Check sheet for the modelled part. Datum: model origin and axes. Units: mm. Face numbers are marked on the shaded views. Give positions to 0.01 mm unless a question says otherwise; leave off trailing zeros.
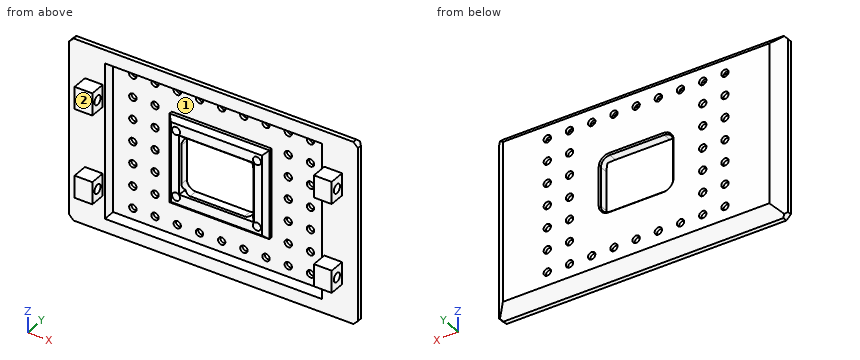
```python
from build123d import *

# Parameters (mm, degrees)
SKETCH1_W           = 130
SKETCH1_H           = 82
BOSS_EXTRUDE1_DEPTH = 2
CHAMFER2_SIZE       = 2
SKETCH4_W           = 8
SKETCH4_H           = 10
BOSS_EXTRUDE2_DEPTH = 7
SKETCH5_R           = 2.05
CUT_EXTRUDE1_DEPTH  = 130.747485656
SKETCH6_W           = 97.8
SKETCH6_H           = 70
CUT_EXTRUDE2_DEPTH  = 5.5
SKETCH7_R           = 1.65
CUT_EXTRUDE3_DEPTH  = 78.860452228
SKETCH10_W          = 50
SKETCH10_H          = 50
BOSS_EXTRUDE3_DEPTH = 1.5
SKETCH11_W          = 45
SKETCH11_H          = 40
BOSS_EXTRUDE4_DEPTH = 3.5
SKETCH12_R          = 1.35
SKETCH12_W          = 32.5
SKETCH12_H          = 25.5
CUT_EXTRUDE4_DEPTH  = 79.115299533
CHAMFER3_SIZE       = 0.6
FILLET1_R           = 4
CHAMFER4_SIZE       = 0.6
SKETCH13_R          = 1.35
BOSS_EXTRUDE5_DEPTH = 1
SKETCH14_R          = 1.8
CUT_EXTRUDE5_DEPTH  = 4
CHAMFER5_SIZE       = 2


with BuildPart() as part:
    # Sketch1 → Boss-Extrude1 (new body)
    with BuildSketch(Plane(origin=(0, 0, 0), x_dir=(1, 0, 0), z_dir=(0, 1, 0))):
        Rectangle(SKETCH1_W, SKETCH1_H)
    extrude(amount=BOSS_EXTRUDE1_DEPTH)

    # Sketch3 → Loft1 section 0
    with BuildSketch(Plane(origin=(0, 7, 0), x_dir=(1, 0, 0), z_dir=(0, 1, 0))):
        with BuildLine():
            Line((-60, -36), (60, -36))
            Line((60, -36), (60, 36))
            Line((60, 36), (-60, 36))
            Line((-60, 36), (-60, -36))
        make_face()
    # Sketch2 → Loft1 section 1
    with BuildSketch(Plane(origin=(0, 2, 0), x_dir=(1, 0, 0), z_dir=(0, 1, 0))):
        with BuildLine():
            Line((65, -41), (65, 41))
            Line((65, 41), (-65, 41))
            Line((-65, 41), (-65, -41))
            Line((-65, -41), (65, -41))
        make_face()
    loft()

    # Chamfer2
    chamfer2_edges = [part.edges().sort_by_distance(p)[0] for p in [
        (65, 1, 41),
        (-65, 1, 41),
        (-65, 1, -41),
        (65, 1, -41),
    ]]
    chamfer(chamfer2_edges, length=CHAMFER2_SIZE)

    # Sketch4 → Boss-Extrude2 (add)
    with BuildSketch(Plane.XZ):
        with Locations((-53.9, 20)):
            Rectangle(SKETCH4_W, SKETCH4_H)
        with Locations((-53.9, -20)):
            Rectangle(SKETCH4_W, SKETCH4_H)
        with Locations((53.9, -20)):
            Rectangle(SKETCH4_W, SKETCH4_H)
        with Locations((53.9, 20)):
            Rectangle(SKETCH4_W, SKETCH4_H)
    extrude(amount=BOSS_EXTRUDE2_DEPTH)

    # Sketch5 → Cut-Extrude1 (cut, through all)
    with BuildSketch(Plane.ZY.offset(57.9)):
        with Locations((-20, -3.5)):
            Circle(SKETCH5_R)
        with Locations((20, -3.5)):
            Circle(SKETCH5_R)
    extrude(amount=-CUT_EXTRUDE1_DEPTH, mode=Mode.SUBTRACT)

    # Sketch6 → Cut-Extrude2 (cut)
    with BuildSketch(Plane.XZ):
        Rectangle(SKETCH6_W, SKETCH6_H)
    extrude(amount=-CUT_EXTRUDE2_DEPTH, mode=Mode.SUBTRACT)

    # Sketch7 → Cut-Extrude3 (cut, through all)
    with BuildSketch(Plane.XZ.offset(-5.5)):
        with Locations(Location((0, 0, 0), (0, 0, 270))):
            Circle(SKETCH7_R)
        with Locations(Location((10, 0, 0), (0, 0, 270))):
            Circle(SKETCH7_R)
        with Locations(Location((20, 0, 0), (0, 0, 270))):
            Circle(SKETCH7_R)
        with Locations(Location((30, 0, 0), (0, 0, 270))):
            Circle(SKETCH7_R)
        with Locations(Location((40, 0, 0), (0, 0, 270))):
            Circle(SKETCH7_R)
        with Locations(Location((10, 10, 0), (0, 0, 270))):
            Circle(SKETCH7_R)
        with Locations(Location((20, 10, 0), (0, 0, 270))):
            Circle(SKETCH7_R)
        with Locations(Location((30, 10, 0), (0, 0, 270))):
            Circle(SKETCH7_R)
        with Locations(Location((40, 10, 0), (0, 0, 270))):
            Circle(SKETCH7_R)
        with Locations(Location((10, 20, 0), (0, 0, 270))):
            Circle(SKETCH7_R)
        with Locations(Location((20, 20, 0), (0, 0, 270))):
            Circle(SKETCH7_R)
        with Locations(Location((30, 20, 0), (0, 0, 270))):
            Circle(SKETCH7_R)
        with Locations(Location((40, 20, 0), (0, 0, 270))):
            Circle(SKETCH7_R)
        with Locations(Location((10, 30, 0), (0, 0, 270))):
            Circle(SKETCH7_R)
        with Locations(Location((20, 30, 0), (0, 0, 270))):
            Circle(SKETCH7_R)
        with Locations(Location((30, 30, 0), (0, 0, 270))):
            Circle(SKETCH7_R)
        with Locations(Location((40, 30, 0), (0, 0, 270))):
            Circle(SKETCH7_R)
        with Locations(Location((0, 10, 0), (0, 0, 270))):
            Circle(SKETCH7_R)
        with Locations(Location((0, 20, 0), (0, 0, 270))):
            Circle(SKETCH7_R)
        with Locations(Location((0, 30, 0), (0, 0, 270))):
            Circle(SKETCH7_R)
        with Locations(Location((-40, 30, 0), (0, 0, 270))):
            Circle(SKETCH7_R)
        with Locations(Location((-30, 30, 0), (0, 0, 270))):
            Circle(SKETCH7_R)
        with Locations(Location((-20, 30, 0), (0, 0, 270))):
            Circle(SKETCH7_R)
        with Locations(Location((-10, 30, 0), (0, 0, 270))):
            Circle(SKETCH7_R)
        with Locations(Location((-40, 20, 0), (0, 0, 270))):
            Circle(SKETCH7_R)
        with Locations(Location((-30, 20, 0), (0, 0, 270))):
            Circle(SKETCH7_R)
        with Locations(Location((-20, 20, 0), (0, 0, 270))):
            Circle(SKETCH7_R)
        with Locations(Location((-10, 20, 0), (0, 0, 270))):
            Circle(SKETCH7_R)
        with Locations(Location((-40, 10, 0), (0, 0, 270))):
            Circle(SKETCH7_R)
        with Locations(Location((-30, 10, 0), (0, 0, 270))):
            Circle(SKETCH7_R)
        with Locations(Location((-20, 10, 0), (0, 0, 270))):
            Circle(SKETCH7_R)
        with Locations(Location((-10, 10, 0), (0, 0, 270))):
            Circle(SKETCH7_R)
        with Locations(Location((-40, 0, 0), (0, 0, 270))):
            Circle(SKETCH7_R)
        with Locations(Location((-30, 0, 0), (0, 0, 270))):
            Circle(SKETCH7_R)
        with Locations(Location((-20, 0, 0), (0, 0, 270))):
            Circle(SKETCH7_R)
        with Locations(Location((-10, 0, 0), (0, 0, 270))):
            Circle(SKETCH7_R)
        with Locations(Location((-10, -10, 0), (0, 0, 270))):
            Circle(SKETCH7_R)
        with Locations(Location((-20, -10, 0), (0, 0, 270))):
            Circle(SKETCH7_R)
        with Locations(Location((-30, -10, 0), (0, 0, 270))):
            Circle(SKETCH7_R)
        with Locations(Location((-40, -10, 0), (0, 0, 270))):
            Circle(SKETCH7_R)
        with Locations(Location((-10, -20, 0), (0, 0, 270))):
            Circle(SKETCH7_R)
        with Locations(Location((-20, -20, 0), (0, 0, 270))):
            Circle(SKETCH7_R)
        with Locations(Location((-30, -20, 0), (0, 0, 270))):
            Circle(SKETCH7_R)
        with Locations(Location((-40, -20, 0), (0, 0, 270))):
            Circle(SKETCH7_R)
        with Locations(Location((-10, -30, 0), (0, 0, 270))):
            Circle(SKETCH7_R)
        with Locations(Location((-20, -30, 0), (0, 0, 270))):
            Circle(SKETCH7_R)
        with Locations(Location((-30, -30, 0), (0, 0, 270))):
            Circle(SKETCH7_R)
        with Locations(Location((-40, -30, 0), (0, 0, 270))):
            Circle(SKETCH7_R)
        with Locations(Location((0, -30, 0), (0, 0, 270))):
            Circle(SKETCH7_R)
        with Locations(Location((0, -20, 0), (0, 0, 270))):
            Circle(SKETCH7_R)
        with Locations(Location((0, -10, 0), (0, 0, 270))):
            Circle(SKETCH7_R)
        with Locations(Location((40, -30, 0), (0, 0, 270))):
            Circle(SKETCH7_R)
        with Locations(Location((30, -30, 0), (0, 0, 270))):
            Circle(SKETCH7_R)
        with Locations(Location((20, -30, 0), (0, 0, 270))):
            Circle(SKETCH7_R)
        with Locations(Location((10, -30, 0), (0, 0, 270))):
            Circle(SKETCH7_R)
        with Locations(Location((40, -20, 0), (0, 0, 270))):
            Circle(SKETCH7_R)
        with Locations(Location((30, -20, 0), (0, 0, 270))):
            Circle(SKETCH7_R)
        with Locations(Location((20, -20, 0), (0, 0, 270))):
            Circle(SKETCH7_R)
        with Locations(Location((10, -20, 0), (0, 0, 270))):
            Circle(SKETCH7_R)
        with Locations(Location((40, -10, 0), (0, 0, 270))):
            Circle(SKETCH7_R)
        with Locations(Location((30, -10, 0), (0, 0, 270))):
            Circle(SKETCH7_R)
        with Locations(Location((20, -10, 0), (0, 0, 270))):
            Circle(SKETCH7_R)
        with Locations(Location((10, -10, 0), (0, 0, 270))):
            Circle(SKETCH7_R)
    extrude(amount=-CUT_EXTRUDE3_DEPTH, mode=Mode.SUBTRACT)

    # Sketch10 → Boss-Extrude3 (add)
    with BuildSketch(Plane(origin=(0, 7, 0), x_dir=(1, 0, 0), z_dir=(0, 1, 0))):
        Rectangle(SKETCH10_W, SKETCH10_H)
    extrude(amount=-BOSS_EXTRUDE3_DEPTH)

    # Sketch11 → Boss-Extrude4 (add)
    with BuildSketch(Plane.XZ.offset(-5.5)):
        Rectangle(SKETCH11_W, SKETCH11_H)
    extrude(amount=BOSS_EXTRUDE4_DEPTH)

    # Sketch12 → Cut-Extrude4 (cut, through all)
    with BuildSketch(Plane(origin=(0, 7, 0), x_dir=(1, 0, 0), z_dir=(0, 1, 0))):
        with Locations(Location((-18.21, 14.785, 0), (0, 0, 270))):
            Circle(SKETCH12_R)
        with Locations(Location((18.21, 14.785, 0), (0, 0, 270))):
            Circle(SKETCH12_R)
        with Locations(Location((18.21, -14.785, 0), (0, 0, 270))):
            Circle(SKETCH12_R)
        with Locations(Location((-18.21, -14.785, 0), (0, 0, 270))):
            Circle(SKETCH12_R)
        Rectangle(SKETCH12_W, SKETCH12_H)
    extrude(amount=-CUT_EXTRUDE4_DEPTH, mode=Mode.SUBTRACT)

    # Chamfer3
    chamfer3_edges = [part.edges().sort_by_distance(p)[0] for p in [
        (0, 2, -12.75),
        (-16.25, 2, 0),
        (0, 2, 12.75),
        (16.25, 2, 0),
    ]]
    chamfer(chamfer3_edges, length=CHAMFER3_SIZE)

    # Fillet1
    fillet1_edges = [part.edges().sort_by_distance(p)[0] for p in [
        (-16.25, 4.8, 12.75),
        (16.25, 4.8, 12.75),
        (16.25, 4.8, -12.75),
        (-16.25, 4.8, -12.75),
    ]]
    fillet(fillet1_edges, radius=FILLET1_R)

    # Chamfer4
    chamfer4_edges = [part.edges().sort_by_distance(p)[0] for p in [
        (16.25, 7, 0),
        (0, 7, 12.75),
        (-16.25, 7, 0),
        (0, 7, -12.75),
        (15.078427125, 7, 11.578427125),
        (-15.078427125, 7, 11.578427125),
        (15.078427125, 7, -11.578427125),
        (-15.078427125, 7, -11.578427125),
    ]]
    chamfer(chamfer4_edges, length=CHAMFER4_SIZE)

    # Sketch13 → Boss-Extrude5 (add)
    with BuildSketch(Plane(origin=(0, 7, 0), x_dir=(1, 0, 0), z_dir=(0, 1, 0))):
        with Locations(Location((-18.21, -14.785, 0), (0, 0, 270))):
            Circle(SKETCH13_R)
        with Locations(Location((18.21, -14.785, 0), (0, 0, 270))):
            Circle(SKETCH13_R)
        with Locations(Location((18.21, 14.785, 0), (0, 0, 270))):
            Circle(SKETCH13_R)
        with Locations(Location((-18.21, 14.785, 0), (0, 0, 270))):
            Circle(SKETCH13_R)
    extrude(amount=-BOSS_EXTRUDE5_DEPTH)

    # Sketch14 → Cut-Extrude5 (cut)
    with BuildSketch(Plane.XZ.offset(-2)):
        with Locations(Location((-18.21, 14.785, 0), (0, 0, 270))):
            Circle(SKETCH14_R)
        with Locations(Location((18.21, 14.785, 0), (0, 0, 270))):
            Circle(SKETCH14_R)
        with Locations(Location((18.21, -14.785, 0), (0, 0, 270))):
            Circle(SKETCH14_R)
        with Locations(Location((-18.21, -14.785, 0), (0, 0, 270))):
            Circle(SKETCH14_R)
    extrude(amount=-CUT_EXTRUDE5_DEPTH, mode=Mode.SUBTRACT)

    # Chamfer5
    chamfer5_edges = [part.edges().sort_by_distance(p)[0] for p in [
        (22.5, 2, 0),
        (0, 2, 20),
        (-22.5, 2, 0),
        (0, 2, -20),
    ]]
    chamfer(chamfer5_edges, length=CHAMFER5_SIZE)


solid = part.part
```
Q1. Sectioned sample at A-A, the plane z = 0. Count the separate pieces of the cut face and the enclosed holes in it, plus the area to 3 significant figures.
Q2. Go/stop test with flat-tipped pins: P1, Ø5.5, axis at x = 30, z = 0, coming from the -Y side; P2, Ø2, axis at y = 3.5, z = -27, coming from the +X side; P3, Ø1, axis at y = -5, z = 22, coming from the +X side; P4, Ø3, axis at x = 0, z = 30, coming from the -Y side. Record where each tip stops, or that it passes through.
Q3. Material ranges on line 1 (X direction, y = 3.5, z = 9); line 2 (X direction, y = 1.25, z = -24); line 3 (Z direction, x = 32, y = 1.25), recorded low to high.
Q4. Draft check along X on the marked faces 1 and 2. Enter one of: pulls with the +X half, pulls with the -X half, needs draft (parallel to the pull), parting line crosses it, or undercut.
Filled in:
1. separate pieces: 6
1. enclosed holes: 0
1. area: 318 mm2
2. P1: stops at y = 5.5
2. P2: stops at x = 64.5
2. P3: stops at x = 57.9
2. P4: passes through
3. line 1: x = -63.5 to -48.9, -22 to -16.24, 16.24 to 22, 48.9 to 63.5
3. line 2: x = -65 to -48.9, 48.9 to 65
3. line 3: z = -41 to -35, 35 to 41
4. face 1: undercut
4. face 2: needs draft
